Geometry: see drawing. Coordinates: mm, zero at the bounding-box minimum. A direction names the side the tool comes from. Give positions to 0.01 mm unless a question says otherwise; leave off trailing zeros. Loops run counter-clockwise (first coordinate to the right, second up) from the corner with the lowest first, then second, coordinate; pieces in that order, holes last. Notation, with made-up numbers: (27, 87.5) -> (61, 87.5) arc R12 cw to (61, 106.5) -> close; hole circle Ø11 at (72, 16). An arc over 180 degrees is marked (long way). One line per question, with ' | ' between items.
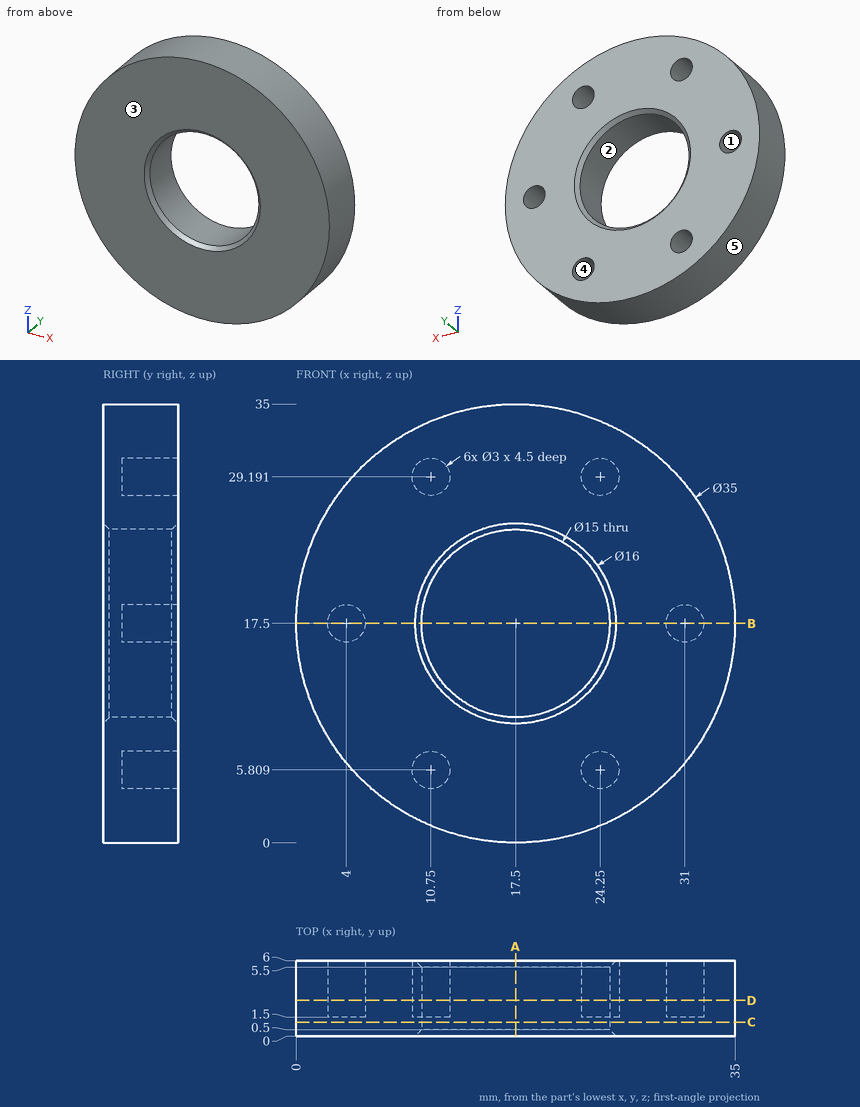
1. Ray query, line 1 along X through (y, z) = (3.1, 17.5); line 2 along Z through (x, y) = (10.75, 2.9) (1 decimal); line 3 along X through (y, z) = (3.75, 5.5). Return the intervals inside material, ascending. Write a range as from..to.
Determined:
line 1: x = 0..2.5, 5.5..10, 25..29.5, 32.5..35 | line 2: z = 1.4..4.3, 7.3..14.2, 20.8..27.7, 30.7..33.6 | line 3: x = 4.76..9.28, 12.22..22.78, 25.72..30.24
2. Section query D-D (y = 2.85). Output: boundary loops of the cut face in (x, z).
Determined:
outline: circle Ø35 at (17.5, 17.5); hole circle Ø3 at (4, 17.5); hole circle Ø3 at (10.75, 5.81); hole circle Ø3 at (10.75, 29.19); hole circle Ø15 at (17.5, 17.5); hole circle Ø3 at (24.25, 5.81); hole circle Ø3 at (24.25, 29.19); hole circle Ø3 at (31, 17.5)
3. Section query A-A (x = 17.5). Output: boundary loops of the cut face in (y, z).
Determined:
outline: (0, 0) -> (6, 0) -> (6, 9.5) -> (5.5, 10) -> (0.5, 10) -> (0, 9.5) -> close; (0, 25.5) -> (0.5, 25) -> (5.5, 25) -> (6, 25.5) -> (6, 35) -> (0, 35) -> close
4. Pin query (flat end, axial travel): P1, Ø1.8, axis at x = 24.25, z = 5.81, coming from the -Y side; P2, Ø2, axis at y = 1.5, z = 19.5, coming from the +X side; P3, Ø3, axis at y = 5.5, z = 14.5, coming from the -X side; P4, Ø2, axis at x = 12, y = 5, coming from the -Z side. Return the tip coordinate at first contact, or that it passes through.
Determined:
P1: stops at y = 0 | P2: stops at x = 34.97 | P3: stops at x = 0.06 | P4: stops at z = 0.59
5. Section query B-B (z = 17.5). Output: boundary loops of the cut face in (x, y).
Determined:
outline: (0, 0) -> (9.5, 0) -> (10, 0.5) -> (10, 5.5) -> (9.5, 6) -> (5.5, 6) -> (5.5, 1.5) -> (2.5, 1.5) -> (2.5, 6) -> (0, 6) -> close; (25, 0.5) -> (25.5, 0) -> (35, 0) -> (35, 6) -> (32.5, 6) -> (32.5, 1.5) -> (29.5, 1.5) -> (29.5, 6) -> (25.5, 6) -> (25, 5.5) -> close
6. Pull-direction query (X, two-part tool) for the marked faces 3, 4 and 5; classes: pulls with the +X half, pulls with the -X half, needs draft (parallel to the pull), parting line crosses it, or undercut.
Determined:
face 3: needs draft | face 4: undercut | face 5: parting line crosses it
7. Section query C-C (y = 1.1). Output: boundary loops of the cut face in (x, z).
Determined:
outline: circle Ø35 at (17.5, 17.5); hole circle Ø15 at (17.5, 17.5)
8. Reachability of the marked faces 1 and 2 from +Z, -Z, +X, -X, +Y, -Y: full face, straight path, thin tool, end or side. Return the list, or none.
Determined:
face 1: +Y | face 2: +Y, -Y
